```python
from build123d import *

# Parameters (mm, degrees)
SKETCH3_R           = 9.25
BOSS_EXTRUDE1_DEPTH = 20


with BuildPart() as part:
    # Sketch3 → Boss-Extrude1 (new body)
    with BuildSketch(Plane(origin=(0, 0, 0), x_dir=(1, 0, 0), z_dir=(0, 1, 0))):
        with BuildLine():
            Line((-41, -11.25), (41, -11.25))
            ThreePointArc((41, -11.25), (52.25, 0), (41, 11.25))
            Line((41, 11.25), (-41, 11.25))
            ThreePointArc((-41, 11.25), (-52.25, 0), (-41, -11.25))
        make_face()
        with Locations((-41, 0)):
            Circle(SKETCH3_R, mode=Mode.SUBTRACT)
        with Locations((-18, 0)):
            Circle(SKETCH3_R, mode=Mode.SUBTRACT)
        with Locations((18, 0)):
            Circle(SKETCH3_R, mode=Mode.SUBTRACT)
        with Locations((41, 0)):
            Circle(SKETCH3_R, mode=Mode.SUBTRACT)
        with BuildLine():
            ThreePointArc((-8.243682204, -6.270576132), (-6.383696467, 0), (-8.243682204, 6.270576132))
            ThreePointArc((-8.243682204, 6.270576132), (-8.325149731, 8.314769866), (-6.567157985, 9.361111111))
            Line((-6.567157985, 9.361111111), (6.982897694, 9.361111111))
            ThreePointArc((6.982897694, 9.361111111), (8.746731902, 8.303920153), (8.645856533, 6.25))
            ThreePointArc((8.645856533, 6.25), (6.75, 0), (8.645856533, -6.25))
            ThreePointArc((8.645856533, -6.25), (8.746731902, -8.303920153), (6.982897694, -9.361111111))
            Line((6.982897694, -9.361111111), (-6.567157985, -9.361111111))
            ThreePointArc((-6.567157985, -9.361111111), (-8.325149731, -8.314769866), (-8.243682204, -6.270576132))
        make_face(mode=Mode.SUBTRACT)
    extrude(amount=BOSS_EXTRUDE1_DEPTH)


solid = part.part
```
The model under review builds one solid part; all positions refer to its coordinate system, in mm. A direction names the side the tool comes from. Round coordinates to 2 decimals unless told otherwise and drop trailing zeros. Order: outer loops, then holes, each group sorted by start corner. A loop starts at its lowest first (then second) coordinate and runs counter-clockwise, first axis right, second up.
(1) For P1, Ø3, axis at y = 11, z = -7.5, coming from the -X side, flat-tipped, find the tip position at first contact; note if it passes through.
Working result:
P1: stops at x = -50.52
(2) Mouldability with a two-part tool opening along X and no side actions: class faces 3 (the face through (0, 10, -9.361)), 4 (the face through (52.247, 9.86, 0.247)), 5 (the face through (-1, 10, 11.25)), 6 (the face through (26.545, 9.86, 3.543)) as released by +X, released by -X, zero draft, split by the parting line, or undercut.
Working result:
face 3: undercut
face 4: released by +X
face 5: zero draft
face 6: undercut
(3) Tool access review of faces 1 (the face through (-8.31, 9.86, 8.34)), 2 (the face through (1, 10, -11.25)): name each direction out of +Z, -Z, +X, -X, +Y, -Y from which nothing blocks a thin tool from reaching the whole face with its end or side.
Working result:
face 1: +Y, -Y
face 2: -Z, +X, -X, +Y, -Y
(4) Take a section at B-B, the plane x = -18. State the section outline as (y, z) points, plus the area to 3 significant figures.
Working result:
outline: (0, -11.25) - (20, -11.25) - (20, -9.25) - (0, -9.25) - close; (0, 9.25) - (20, 9.25) - (20, 11.25) - (0, 11.25) - close
area: 80.0 mm2
(5) Take a section at C-C, the plane y = 9.5. State the section outline as (x, z) points.
Working result:
outline: (-41, -11.25) - (41, -11.25) arc R11.25 ccw to (41, 11.25) - (-41, 11.25) arc R11.25 ccw to start; hole circle Ø18.5 at (-41, 0); hole circle Ø18.5 at (-18, 0); hole (-8.24, -6.27) arc R2 ccw to (-6.57, -9.36) - (6.98, -9.36) arc R2 ccw to (8.65, -6.25) arc R11.25 cw to (8.65, 6.25) arc R2 ccw to (6.98, 9.36) - (-6.57, 9.36) arc R2 ccw to (-8.24, 6.27) arc R11.5 cw to start; hole circle Ø18.5 at (18, 0); hole circle Ø18.5 at (41, 0)
(6) Take a section at D-D, the plane z = -4. State the section outline as (x, y) points, plus the area to 3 significant figures.
Working result:
outline: (-51.51, 0) - (-49.34, 0) - (-49.34, 20) - (-51.51, 20) - close; (-32.66, 0) - (-26.34, 0) - (-26.34, 20) - (-32.66, 20) - close; (-9.66, 0) - (-7.1, 0) - (-7.1, 20) - (-9.66, 20) - close; (7.49, 0) - (9.66, 0) - (9.66, 20) - (7.49, 20) - close; (26.34, 0) - (32.66, 0) - (32.66, 20) - (26.34, 20) - close; (49.34, 0) - (51.51, 0) - (51.51, 20) - (49.34, 20) - close
area: 434 mm2
(7) Wall thickness on L1, parallel to Z at x = -41, y = 14.25; L2, parallel to X at y = 15.5, z = 2.5; L3, parallel to Z at x = 38, y = 17.75: over which ranges is each line inside the solid? List them lowest first.
Working result:
L1: z = -11.25 to -9.25, 9.25 to 11.25
L2: x = -51.97 to -49.91, -32.09 to -26.91, -9.09 to -6.66, 7.03 to 9.09, 26.91 to 32.09, 49.91 to 51.97
L3: z = -11.25 to -8.75, 8.75 to 11.25
(8) Take a section at A-A, the plane z = 0. State the section outline as (x, y) points, plus the area to 3 significant figures.
Working result:
outline: (-52.25, 0) - (-50.25, 0) - (-50.25, 20) - (-52.25, 20) - close; (-31.75, 0) - (-27.25, 0) - (-27.25, 20) - (-31.75, 20) - close; (-8.75, 0) - (-6.38, 0) - (-6.38, 20) - (-8.75, 20) - close; (6.75, 0) - (8.75, 0) - (8.75, 20) - (6.75, 20) - close; (27.25, 0) - (31.75, 0) - (31.75, 20) - (27.25, 20) - close; (50.25, 0) - (52.25, 0) - (52.25, 20) - (50.25, 20) - close
area: 347 mm2
